Job drawing, mm, ordinate dimensions from the low corner. One solid piece. Coordinates: 2 decimals unless noted, no trailing zeros. Order: outer loops, then holes, each group sorted by start corner. A loop starts at its lowest first (then second) coordinate and runs counter-clockwise, first axis right, second up. Notation, with made-up numbers: (48, 73) - (107, 73) arc R26 cw to (107, 101) - close; hole circle Ø5 at (-23.75, 53.5). An arc over 180 degrees is marked (long way). Return JSON: item names as keys, results as strings.
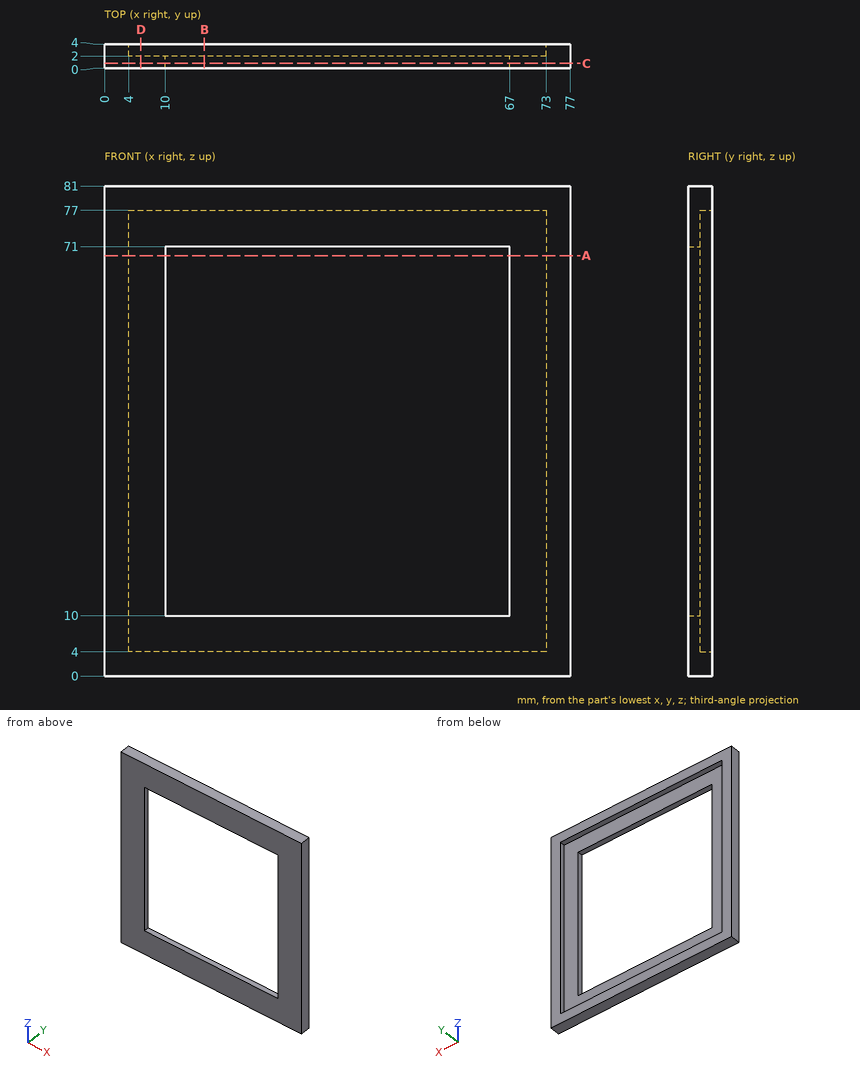
1. Cut at A-A on z = 69.5. Give the cut face in (x, y), plus the area to 3 significant figures.
Check values:
{"outline": "(0, 0) - (10, 0) - (10, 2) - (4, 2) - (4, 4) - (0, 4) - close; (67, 0) - (77, 0) - (77, 4) - (73, 4) - (73, 2) - (67, 2) - close", "area": "56.0 mm²"}
2. Probe L1, parallel to X at y = 3.3, z = 68.5; L2, parallel to Z at x = 18, y = 2.25; L3, parallel to Z at x = 13, y = 0.55. List the from-to ranges inside material, lowest first.
Check values:
{"L1": "0 to 4, 73 to 77", "L2": "0 to 4, 77 to 81", "L3": "0 to 10, 71 to 81"}
3. Cut at B-B on x = 16.5. Give the cut face in (y, z).
Check values:
{"outline": "(0, 0) - (4, 0) - (4, 4) - (2, 4) - (2, 10) - (0, 10) - close; (0, 71) - (2, 71) - (2, 77) - (4, 77) - (4, 81) - (0, 81) - close"}
4. Cut at D-D on x = 6. Give the cut face in (y, z).
Check values:
{"outline": "(0, 0) - (4, 0) - (4, 4) - (2, 4) - (2, 77) - (4, 77) - (4, 81) - (0, 81) - close"}
5. Drop a flat-ended pin along its axis: pin 1 (3 mm diameter, centred on x = 9, z = 10.5, fed in from +Y). Give the stop position or say it passes through.
Check values:
{"pin 1": "y = 2"}
6. Cut at C-C on y = 0.8. Give the cut face in (x, z).
Check values:
{"outline": "(0, 0) - (77, 0) - (77, 81) - (0, 81) - close; hole (10, 10) - (67, 10) - (67, 71) - (10, 71) - close"}
